The listing builds one solid part. Answer for the finished solid, in the listing's coordinates (mm). A direction names the side the tool comes from. Give positions to 0.01 mm unless a question says otherwise; leave off trailing zeros. Write each loop counter-clockwise with the first axis right and the second up, starting at its lowest first coordinate (ties: lowest second). Pieces come first, ordered by that corner, then holes. Notation, with made-up numbers: M -19,25 L 24,25 A20 ccw 24,50 Z; hole C 65.25,-12.5 d5. An arc over 180 degrees is marked long. Answer as a JSON object with one key per item and string values.
```python
from build123d import *

# Parameters (mm, degrees)
SKETCH1_R           = 22
SKETCH1_R_2         = 16
BOSS_EXTRUDE1_DEPTH = 6
BOSS_EXTRUDE2_DEPTH = 6
CUT_EXTRUDE1_DEPTH  = 37.933063475
SKETCH4_W           = 6
SKETCH4_H           = 30
BOSS_EXTRUDE3_DEPTH = 6
CUT_EXTRUDE2_DEPTH  = 55.497937543
FILLET1_R           = 10
FILLET2_R           = 10
SKETCH6_W           = 6
SKETCH6_H           = 30
BOSS_EXTRUDE4_DEPTH = 6
FILLET3_R           = 4


with BuildPart() as part:
    # Sketch1 → Boss-Extrude1 (new body)
    with BuildSketch(Plane(origin=(0, 0, 0), x_dir=(0, 0, -1), z_dir=(1, 0, 0))):
        Circle(SKETCH1_R)
        Circle(SKETCH1_R_2, mode=Mode.SUBTRACT)
    extrude(amount=BOSS_EXTRUDE1_DEPTH)

    # Sketch2 → Boss-Extrude2 (add)
    with BuildSketch(Plane(origin=(6, 0, 0), x_dir=(0, 0, -1), z_dir=(1, 0, 0))):
        Polygon((19.052558883, 11), (29.052558883, -6.320508076), (23.856406461, -9.320508076), (13.856406461, 8), align=None)
    extrude(amount=-BOSS_EXTRUDE2_DEPTH)

    # Sketch3 → Cut-Extrude1 (cut, through all)
    with BuildSketch(Plane(origin=(6, 0, 0), x_dir=(0, 0, -1), z_dir=(1, 0, 0))):
        with BuildLine():
            ThreePointArc((16, 0), (12.693653445, -9.740182864), (4.141104722, -15.454813221))
            Line((4.141104722, -15.454813221), (5.694018992, -21.250368178))
            ThreePointArc((5.694018992, -21.250368178), (15.779826764, -15.329614062), (21.406240896, -5.076696831))
            Line((21.406240896, -5.076696831), (13.856406461, 8))
            ThreePointArc((13.856406461, 8), (15.454813221, 4.141104722), (16, 0))
        make_face()
    extrude(amount=-CUT_EXTRUDE1_DEPTH, mode=Mode.SUBTRACT)

    # Sketch4 → Boss-Extrude3 (add)
    with BuildSketch(Plane(origin=(6, 0, 0), x_dir=(0, 0, -1), z_dir=(1, 0, 0))):
        with Locations((0, -30.716233646)):
            Rectangle(SKETCH4_W, SKETCH4_H)
    extrude(amount=-BOSS_EXTRUDE3_DEPTH)

    # Sketch5 → Cut-Extrude2 (cut, through all)
    with BuildSketch(Plane(origin=(6, 0, 0), x_dir=(0, 0, -1), z_dir=(1, 0, 0))):
        with BuildLine():
            Line((3, -21.794494718), (3, -15.716233646))
            Line((3, -15.716233646), (4.141104722, -15.454813221))
            Line((4.141104722, -15.454813221), (5.694018992, -21.250368178))
            ThreePointArc((5.694018992, -21.250368178), (4.374209957, -21.657103353), (3, -21.794494718))
        make_face()
    extrude(amount=-CUT_EXTRUDE2_DEPTH, mode=Mode.SUBTRACT)

    # Fillet1
    # the kernel refuses this fillet: 10 mm, written as the material it adds along each edge
    with BuildSketch(Plane(origin=(6, -21.794494718, 3), x_dir=(0, -1, 0), z_dir=(-1, 0, 0))) as fillet1_piece_1:
        with BuildLine():
            CenterArc((7.445888317, 10), FILLET1_R, 203.969482318, 66.030517682)
            ThreePointArc((-1.691731382, 5.9375), (-0.636552127, 3.028388286), (0, 0))
            Line((0, 0), (7.445888317, 0))
        make_face()
    extrude(amount=6)
    # the kernel refuses this fillet: 10 mm, written as the material it takes off along each edge
    with BuildSketch(Plane(origin=(28.912878475, -15.716233646, -3), x_dir=(0, -1, 0), z_dir=(-1, 0, 0))) as fillet1_2_piece_1:
        with BuildLine():
            CenterArc((9.16515139, 10), FILLET1_R, 203.578178478, 66.421821522)
            Line((0, 6), (0, 0))
            Line((0, 0), (9.16515139, 0))
        make_face()
    extrude(amount=51.82575695, mode=Mode.SUBTRACT)

    # Fillet2
    fillet2_edges = [part.edges().sort_by_distance(p)[0] for p in [
        (3, -15.716233646, 3),
    ]]
    fillet(fillet2_edges, radius=FILLET2_R)

    # Sketch6 → Boss-Extrude4 (add)
    with BuildSketch(Plane.ZY):
        Polygon((27.04163056, -43.189321711), (3, -67.230952271), (3, -75.716233646), (31.284271247, -47.431962398), align=None)
        with Locations((0, -60.716233646)):
            Rectangle(SKETCH6_W, SKETCH6_H)
    boss_extrude4 = extrude(amount=-BOSS_EXTRUDE4_DEPTH)

    # Mirror1: Boss-Extrude4 across plane
    add(boss_extrude4.mirror(Plane.XY))

    # Fillet3
    fillet3_edges = [part.edges().sort_by_distance(p)[0] for p in [
        (3, -75.716233646, 3),
        (3, -75.716233646, -3),
        (3, -67.230952271, 3),
        (3, -67.230952271, -3),
    ]]
    fillet(fillet3_edges, radius=FILLET3_R)


solid = part.part
```
1. Consider line 1 along Z through (x, y) = (2.5, -54); line 2 along Z through (x, y) = (1.25, -44.5); line 3 along Y through (x, z) = (4.75, 13.5). Determine where each line is inside the solid, lowest interval first.
Verdict:
{"line 1": "z = -24.72 to -16.23, -3 to 3, 16.23 to 24.72", "line 2": "z = -28.35 to -25.73, -3 to 3, 25.73 to 28.35", "line 3": "y = -65.22 to -56.73, -17.37 to -8.59, 8.59 to 17.37"}
2. For faces 1 (the flat face through (2.96, -45.34, -29.19)), 2 (the flat face through (6, -27, 0)), 3 (the flat face through (3, -44, 3)), 4 (the cylindrical face through (3.04, -23.72, 4.66)), 5 (the flat face through (3.042, 2.461, -23.983)), determine the directions among +Z, -Z, +X, -X, +Y, -Y from which every point of the face is accessible in a straight line to the end or side of a thin tool.
Verdict:
{"face 1": "-Z, +X, -X", "face 2": "+Z, -Z, +X, +Y, -Y", "face 3": "+X, -X", "face 4": "+Z, +X, -X", "face 5": "-Z, +X, -X, +Y"}
3. Flat-ended cylindrical pins translate along their axes: pin 1 (1.5 mm diameter, centred on x = 1.5, z = 16, fed in from +Y); pin 2 (3 mm diameter, centred on x = 1.5, z = 7, fed in from +Y); pin 3 (1.5 mm diameter, centred on x = 2.5, y = -15.5, fed in from -Z). Find the tip coordinate at first contact, or state that the pin passes through.
Verdict:
{"pin 1": "stops at y = 15.86", "pin 2": "stops at y = 21.3", "pin 3": "stops at z = 2.23"}
4. A cutting plane is placed at B-B, the plane z = 19. Give the vertices of the cut face in (x, y), plus the area to 3 significant figures.
Verdict:
{"outline": "M 0,-59.72 L 6,-59.72 L 6,-51.23 L 0,-51.23 Z; M 0,-11.09 L 6,-11.09 L 6,11.09 L 0,11.09 Z", "area": "184 mm2"}
5. The mould has two halves that part along Y. Classify faces 6 (the cylindrical face through (3, 15.1, 16)), 7 (the flat face through (2.958, -61.178, -17.538)), 8 (the flat face through (2.96, -45.34, 29.19)): released by +Y, released by -Y, zero draft, split by the parting line, or undercut.
Verdict:
{"face 6": "undercut", "face 7": "released by -Y", "face 8": "released by +Y"}
6. A cutting plane is placed at A-A, the plane y = 0. Give the vertices of the cut face in (x, z), plus the area to 3 significant figures.
Verdict:
{"outline": "M 0,-25.4 L 6,-25.4 L 6,-18.48 L 0,-18.48 Z; M 0,16 L 6,16 L 6,22 L 0,22 Z", "area": "77.6 mm2"}
7. A cutting plane is placed at C-C, the plane y = -68.5. Give the vertices of the cut face in (x, z).
Verdict:
{"outline": "M 0,-10.22 L 6,-10.22 L 6,10.22 L 0,10.22 Z"}
